Can you work these out from the model? Positions are in its coordinate system, mm. A direction names the side the tool comes from. Give positions to 0.01 mm unless a question says otherwise; leave off trailing zeros. Order: outer loops, then holes, each group sorted by start corner. A loop starts at its lowest first (then second) coordinate and runs counter-clockwise, first axis right, second up. Notation, with made-up numbers: M 21.5,-5.5 L 78.5,-5.5 A18 ccw 78.5,22.5 Z; hole C -5.5,-1 d8. An arc over 180 degrees is marked long. Write each question's results on one line, items separated by ' | '.
from build123d import *

# Parameters (mm, degrees)
CUT_EXTRUDE_1_DEPTH = 1


with BuildPart() as part:
    # 草图4 → 旋转1 (revolve)
    with BuildSketch(Plane(origin=(0, 0, 0), x_dir=(1, 0, 0), z_dir=(0, 1, 0)), mode=Mode.PRIVATE) as revolve_1_sk:
        Polygon((0, 0), (0, 2.75), (2, 1.5), (12, 1.5), (12, 0), align=None)
    revolve(revolve_1_sk.sketch.rotate(Axis((-2.103529412, 0, 0), (1, 0, 0)), 180), axis=Axis((-2.103529412, 0, 0), (1, 0, 0)))

    # 草图5 → 切除-拉伸1 (cut)
    with BuildSketch(Plane.ZY):
        Polygon((-0.25, 0.25), (-1.25, 0.25), (-1.25, -0.25), (-0.25, -0.25), (-0.25, -1.25), (0.25, -1.25), (0.25, -0.25), (1.25, -0.25), (1.25, 0.25), (0.25, 0.25), (0.25, 1.25), (-0.25, 1.25), align=None)
    extrude(amount=-CUT_EXTRUDE_1_DEPTH, mode=Mode.SUBTRACT)


solid = part.part
(1) For faces 1 (the face through (0.5, -0.25, 0.7)), 2 (the face through (12, 0, 0)), which set-ups out of +Z, -Z, +X, -X, +Y, -Y let a thin tool reach every point of the face, with its end or its side?
Data:
face 1: -X | face 2: +Z, -Z, +X, +Y, -Y
(2) I need wall thicknesses on L1, parallel to X at y = 1.8, z = -0.2; L2, parallel to Z at x = 2.75, y = 0.1; L3, parallel to X at y = 0, z = -0.3. Which ranges of each line are inside material? Lowest first, please. Write a range as from..to.
Data:
L1: x = 0..1.5 | L2: z = -1.5..1.5 | L3: x = 1..12
(3) Imagine slicing it at A-A, the plane z = 0. Write out the boundary of the cut face in (x, y), plus the area to 3 significant figures.
Data:
outline: M 0,-2.75 L 2,-1.5 L 12,-1.5 L 12,1.5 L 2,1.5 L 0,2.75 L 0,1.25 L 1,1.25 L 1,-1.25 L 0,-1.25 Z | area: 36.0 mm2
(4) We'd pull the mould along Z, two halves only. Please class faces 3 (the face through (1, 0, 0)), 4 (the face through (7.07, -0.45, 1.43)), 5 (the face through (0, 1, -1)): +Z half, -Z half, draft (parallel to the pull), parting line (faces both ways), or undercut.
Data:
face 3: undercut | face 4: parting line | face 5: draft
(5) Will these pins go through, and if not, where does the flat tip stop? P1, Ø0.8, axis at x = 0.5, z = -1, coming from the +Y side; P2, Ø2, axis at x = 11, y = -1, coming from the -Z side; P3, Ø1.5, axis at x = 2, z = 2, coming from the +Y side.
Data:
P1: stops at y = 2.53 | P2: stops at z = -1.5 | P3: stops at y = 1.1
(6) Imagine slicing it at D-D, the plane x = 1.5. Write out the boundary of the cut face in (y, z) (1 decimal).
Data:
outline: C 0,0 d3.6
(7) Imagine slicing it at C-C, the plane x = 4. Write out the boundary of the cut face in (y, z).
Data:
outline: C 0,0 d3
